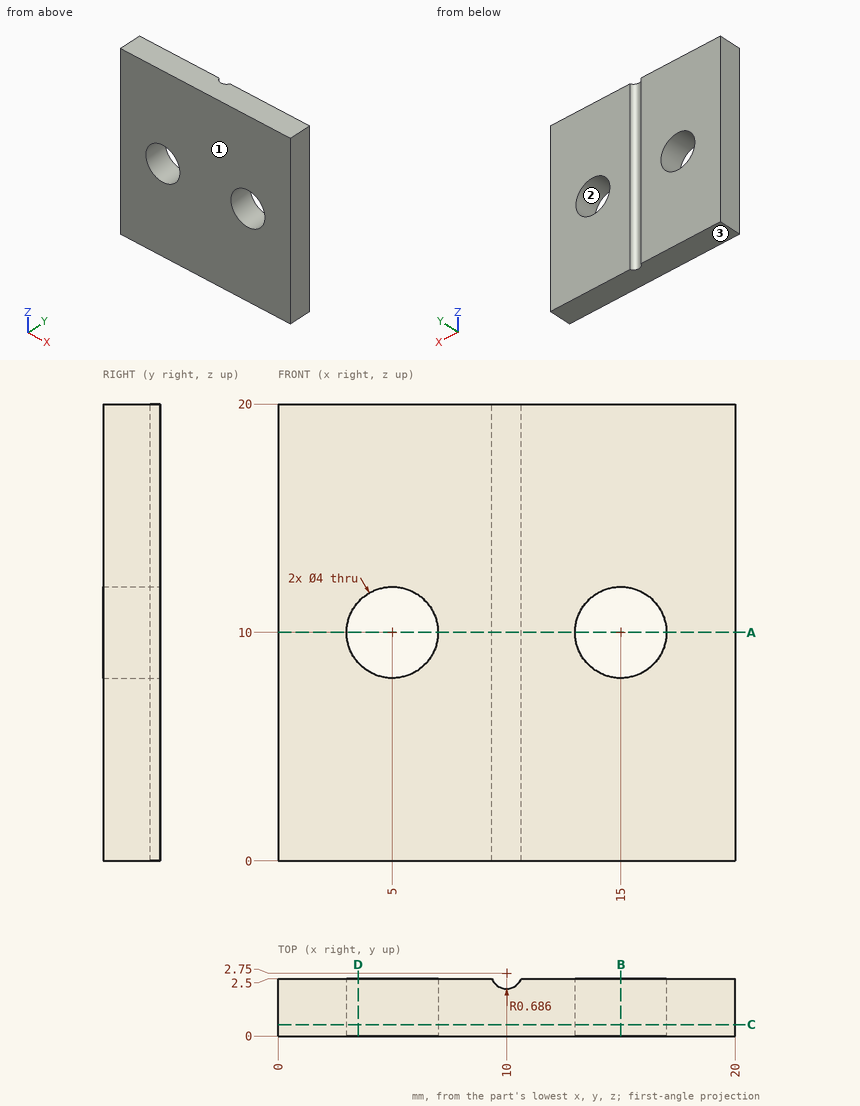
Drawing for the job (mm, zero at the part's lowest x, y, z). Coordinates: 2 decimals unless noted, no trailing zeros. Order: outer loops, then holes, each group sorted by start corner. A loop starts at its lowest first (then second) coordinate and runs counter-clockwise, first axis right, second up. Notation, with made-up numbers: (37, 57.5) -> (63, 57.5) arc R17 ccw to (63, 64.5) -> close; hole circle Ø3 at (-13, -29). An arc over 180 degrees is marked (long way). One line per item, written item: value.
(1) Slice it at B-B, the plane x = 15. List the corners of the cut face in (y, z).
Checked values:
outline: (0, 0) -> (2.5, 0) -> (2.5, 8) -> (0, 8) -> close; (0, 12) -> (2.5, 12) -> (2.5, 20) -> (0, 20) -> close
(2) Slice it at D-D, the plane x = 3.5. List the corners of the cut face in (y, z), plus the area to 3 significant figures.
Checked values:
outline: (0, 0) -> (2.5, 0) -> (2.5, 8.68) -> (0, 8.68) -> close; (0, 11.32) -> (2.5, 11.32) -> (2.5, 20) -> (0, 20) -> close
area: 43.4 mm2
(3) Slice it at A-A, the plane z = 10. List the corners of the cut face in (x, y).
Checked values:
outline: (0, 0) -> (3, 0) -> (3, 2.5) -> (0, 2.5) -> close; (7, 0) -> (13, 0) -> (13, 2.5) -> (10.64, 2.5) arc R0.69 cw to (9.36, 2.5) -> (7, 2.5) -> close; (17, 0) -> (20, 0) -> (20, 2.5) -> (17, 2.5) -> close
(4) Probe line 1 (X direction, y = 2, z = 10); line 2 (Z direction, x = 5, y = 0.85); line 3 (X direction, y = 1.1, z = 8.5). List the from-to ranges inside material, lowest first. Write a range as [from, to].
Checked values:
line 1: [0, 3], [7, 13], [17, 20]
line 2: [0, 8], [12, 20]
line 3: [0, 3.68], [6.32, 13.68], [16.32, 20]
(5) Mould opens along Z. For the marked faces 1, 2 and 3 say: pulls with the +Z half, pulls with the -Z half, needs draft (parallel to the pull), parting line crosses it, or undercut.
Checked values:
face 1: needs draft
face 2: undercut
face 3: pulls with the -Z half
(6) Slice it at C-C, the plane y = 0.5. List the corners of the cut face in (x, z), plus the area to 3 significant figures.
Checked values:
outline: (0, 0) -> (20, 0) -> (20, 20) -> (0, 20) -> close; hole circle Ø4 at (5, 10); hole circle Ø4 at (15, 10)
area: 375 mm2
